For this review, take the finished solid that the model builds, in its own axes (mm). Round coordinates to 2 decimals unless told otherwise and drop trailing zeros. Order: outer loops, then holes, each group sorted by start corner. A loop starts at its lowest first (then second) coordinate and runs counter-clockwise, first axis right, second up.
from build123d import *

# Parameters (mm, degrees)
SKETCH1_R           = 7
SKETCH1_R_2         = 4
BOSS_EXTRUDE1_DEPTH = 15
SKETCH2_R           = 5
BOSS_EXTRUDE2_DEPTH = 700
CHAMFER1_SIZE       = 2


with BuildPart() as part:
    # Sketch1 → Boss-Extrude1 (new body)
    with BuildSketch(Plane(origin=(0, 0, 0), x_dir=(1, 0, 0), z_dir=(0, 1, 0))):
        with Locations(Location((0, 0, 0), (0, 0, 270))):
            Circle(SKETCH1_R)
        with Locations(Location((0, 0, 0), (0, 0, 270))):
            Circle(SKETCH1_R_2, mode=Mode.SUBTRACT)
    extrude(amount=BOSS_EXTRUDE1_DEPTH)

    # Sketch2 → Boss-Extrude2 (add)
    with BuildSketch(Plane.XZ):
        with Locations(Location((0, 0, 0), (0, 0, 90))):
            Circle(SKETCH2_R)
    extrude(amount=BOSS_EXTRUDE2_DEPTH)

    # Chamfer1
    chamfer1_edges = [part.edges().sort_by_distance(p)[0] for p in [
        (0, 0, -5),
    ]]
    chamfer(chamfer1_edges, length=CHAMFER1_SIZE - 0.0001)  # a hair under: the kernel refuses the full size


solid = part.part
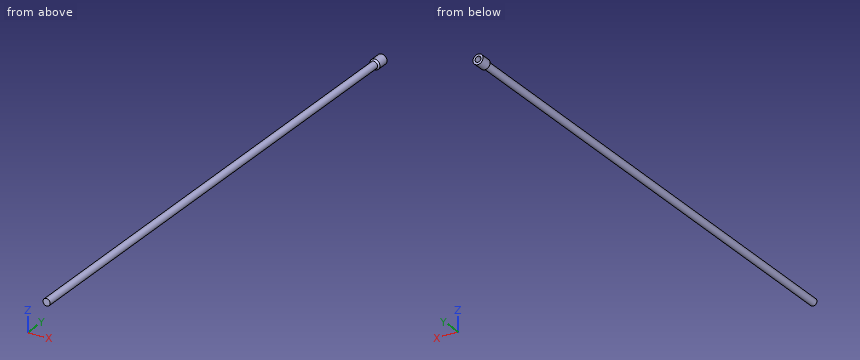
(1) Clearance check with flat-ended pins moving along their axes: P1, Ø2, axis at x = 5.5, z = 2.5, coming from the -Y side; P2, Ø2, axis at x = -4.5, y = -154, coming from the -Z side; P3, Ø5, axis at y = -210, z = -4.5, coming from the +X side. State where each tip first meets the part, or that it passes through.
(2) Add section C-C on y = -515.5. Give the boundary of the cut face in (x, z).
(3) Wall thickness on L1, parallel to X at y = 10.5, z = 0; L2, parallel to Y at x = -1.75, z = -1.25; L3, parallel to Y at x = 2.25, z = -6.5: over which ranges is each line inside the solid? List them lowest first.
Here are the results:
1. P1: stops at y = -1.96
1. P2: stops at z = -3.57
1. P3: stops at x = 4.58
2. outline: circle Ø10 at (0, 0)
3. L1: x = -7 to -4, 4 to 7
3. L2: y = -700 to 0
3. L3: y = -0.12 to 15
